```python
from build123d import *

# Parameters (mm, degrees)
F0_W     = 112
F0_H     = 87
F0_R     = 1.5
F1_DEPTH = 2
F2_R     = 2
F3_W     = 10
F3_H     = 15
F3_R     = 3.5
F4_DEPTH = 2.001


with BuildPart() as f1:
    # F0 (on Top) → F1 (new body)
    with BuildSketch(Plane.XY):
        Rectangle(F0_W, F0_H)
        with Locations((-52.25, -39.75)):
            Circle(F0_R, mode=Mode.SUBTRACT)
        with Locations((52.25, -39.75)):
            Circle(F0_R, mode=Mode.SUBTRACT)
        with Locations((-52.25, 39.75)):
            Circle(F0_R, mode=Mode.SUBTRACT)
        with Locations((52.25, 39.75)):
            Circle(F0_R, mode=Mode.SUBTRACT)
    extrude(amount=F1_DEPTH)

    # F2
    f2_edges = [f1.edges().sort_by_distance(p)[0] for p in [
        (-56, -43.5, 1),
        (-56, 43.5, 1),
        (56, 43.5, 1),
        (56, -43.5, 1),
    ]]
    fillet(f2_edges, radius=F2_R)

    # F3 (on face) → F4 (cut, through all)
    with BuildSketch(Plane.XY.offset(2)):
        with Locations((-44.25, 36)):
            Rectangle(F3_W, F3_H)
        with Locations((-34.5, 37.2)):
            Circle(F3_R)
    extrude(amount=-F4_DEPTH, mode=Mode.SUBTRACT)


solid = f1.part
```
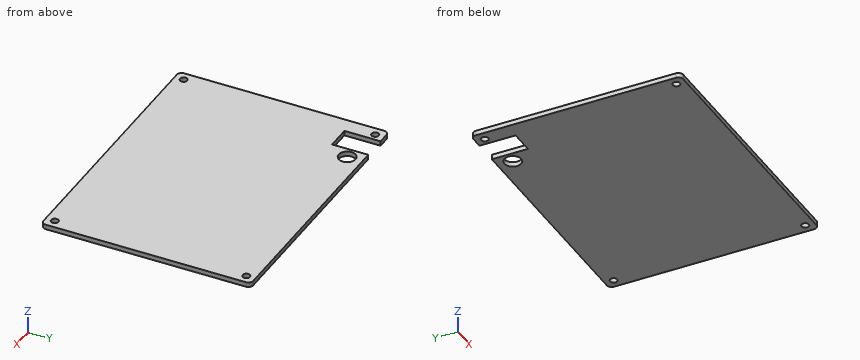
CAD build for the part. Positions are in the model's coordinates, mm. Give positions to 0.01 mm unless a question says otherwise; leave off trailing zeros. Loops run counter-clockwise (first coordinate to the right, second up) from the corner with the lowest first, then second, coordinate; pieces in that order, holes last. Notation, with made-up numbers: M -37,69.5 L -18,69.5 A17 ccw -18,82.5 Z; hole C -39,89 d8. An arc over 180 degrees is marked long. Use one line per item in the form item = value.
Item 1: Slice it at C-C (z = 0.9). List the corners of the cut face in (x, y), plus the area to 3 significant figures.
Determined:
outline = M -56,-41.5 A2 ccw -54,-43.5 L 54,-43.5 A2 ccw 56,-41.5 L 56,41.5 A2 ccw 54,43.5 L -39.25,43.5 L -39.25,28.5 L -49.25,28.5 L -49.25,43.5 L -54,43.5 A2 ccw -56,41.5 Z; hole C -52.25,-39.75 d3; hole C -52.25,39.75 d3; hole C -34.5,37.2 d7; hole C 52.25,-39.75 d3; hole C 52.25,39.75 d3
area = 9,520 mm2
Item 2: Slice it at A-A (y = -39.75). List the corners of the cut face in (x, z).
Determined:
outline = M -56,0 L -53.75,0 L -53.75,2 L -56,2 Z; M -50.75,0 L 50.75,0 L 50.75,2 L -50.75,2 Z; M 53.75,0 L 56,0 L 56,2 L 53.75,2 Z
Item 3: Drill centre lines: probe 1 along Y at (x, z) = (52.25, 1.5); probe 2 along X at (y, z) = (-38.5, 0.5); probe 3 along X at (y, z) = (35, 0.7). Where is each one in solid material? Low to high. Write a range as from..to.
Determined:
probe_1 = -43.5..-41.25, -38.25..38.25, 41.25..43.5
probe_2 = -56..-53.08, -51.42..51.42, 53.08..56
probe_3 = -56..-49.25, -39.25..-37.22, -31.78..56
Item 4: Slice it at B-B (x = -52.25). List the corners of the cut face in (y, z), plus the area to 3 significant figures.
Determined:
outline = M -43.5,0 L -41.25,0 L -41.25,2 L -43.5,2 Z; M -38.25,0 L 38.25,0 L 38.25,2 L -38.25,2 Z; M 41.25,0 L 43.5,0 L 43.5,2 L 41.25,2 Z
area = 162 mm2
Item 5: Slice it at D-D (x = -34.5). List the corners of the cut face in (y, z), plus the area to 3 significant figures.
Determined:
outline = M -43.5,0 L 33.7,0 L 33.7,2 L -43.5,2 Z; M 40.7,0 L 43.5,0 L 43.5,2 L 40.7,2 Z
area = 160 mm2
Item 6: Flat gauge pin, fed straight in: pin 1 (1 mm diameter, centred on x = -45, z = 1.5, fed in from +Y). Where does the tip first touch, or does it go through?
Determined:
pin_1 = 28.5
